from build123d import *

# Parameters (mm, degrees)
F1_DEPTH = 25


# Not quite as in the source:
# - a feature names something its author has since deleted; it is built from what else it names


with BuildPart() as f1:
    # F0 (on Top) → F1 (new body)
    with BuildSketch(Plane.XY):
        with BuildLine():
            Line((12.25, 5.25), (12.25, -5.25))
            Line((12.25, -5.25), (17.25, -5.25))
            Line((17.25, -5.25), (17.25, 10.25))
            Line((17.25, 10.25), (-17.288029389, 10.25))
            add(Edge.make_bspline(
                [(-17.288029389, 10.25), (-33.9326616892, 3.4588538136), (-27.6432598671, -11.5939724111), (-20.8629015828, -23.4088676175)],
                knots=[0, 0, 0, 0, 33.6081495202, 33.6081495202, 33.6081495202, 33.6081495202], degree=3))
            ThreePointArc((-20.8629015828, -23.4088676175), (-18.8330680728, -21.5504075494), (-16.1829780698, -20.8080323883))
            ThreePointArc((-16.1829780698, -20.8080323883), (-15.6956355504, -20.8090410674), (-15.2100205721, -20.8500513288))
            Line((-15.2100205721, -20.8500513288), (-15.2100205721, 3.0333888489))
            Line((-15.2100205721, 3.0333888489), (-12.4874287694, 3.0333888489))
            Line((-12.4874287694, 3.0333888489), (-12.25, 5.25))
            Line((-12.25, 5.25), (12.25, 5.25))
        make_face()
        Polygon((-12.4874287694, 3.0333888489), (-12.25, 3.0333888489), (-12.25, 5.25), align=None)
        with BuildLine():
            ThreePointArc((-10.0197441457, -26.7353467643), (-10.6063091532, -24.1634313379), (-12.25, -22.1001601804))
            ThreePointArc((-12.25, -22.1001601804), (-13.5686599523, -21.3031901955), (-15.0480940947, -20.872725511))
            Line((-15.0480940947, -20.872725511), (-15.2100205721, -22.3844548448))
            Line((-15.2100205721, -22.3844548448), (-15.2100205721, -20.8500513288))
            ThreePointArc((-15.2100205721, -20.8500513288), (-15.6956355504, -20.8090410674), (-16.1829780698, -20.8080323883))
            ThreePointArc((-16.1829780698, -20.8080323883), (-18.8330680728, -21.5504075494), (-20.8629015828, -23.4088676175))
            ThreePointArc((-20.8629015828, -23.4088676175), (-17.691321516, -32.4063150838), (-10.0197441457, -26.7353467643))
        make_face()
    extrude(amount=F1_DEPTH)


solid = f1.part
Can you work these out from the model? Positions are in its coordinate system, mm. A direction names the side the tool comes from. Give positions to 0.01 mm unless a question says otherwise; leave off trailing zeros. Order: outer loops, then holes, each group sorted by start corner. A loop starts at its lowest first (then second) coordinate and runs counter-clockwise, first axis right, second up. Notation, with made-up numbers: M 13,11 L 51,11 A24 cw 51,21 Z; hole C 26,-24 d11. An arc over 180 degrees is marked long. One line per question, with ' | ' between items.
Item 1: I'm going to push flat-ended pins straight in: pin 1 Ø0.9 at (x, z) = (-14, 11) entering from -Y; pin 2 Ø10 at (x, y) = (-12.5, -5.5) entering from -Z; pin 3 Ø2.5 at (x, z) = (14.5, 9) entering from -Y; pin 4 Ø4 at (y, z) = (-23.5, 3) entering from +X. Where does each tip first touch, or does it pass through?
Answer block:
pin 1: stops at y = -32.47 | pin 2: stops at z = 0 | pin 3: stops at y = -5.25 | pin 4: stops at x = -10.15
Item 2: Suppose I cut it at B-B, the plane x = 8. Write out the boundary of the cut face in (y, z).
Answer block:
outline: M 5.25,0 L 10.25,0 L 10.25,25 L 5.25,25 Z
Item 3: We'd pull the mould along X, two halves only. Please class faces 1 (the face through (15, -5.25, 12)), 2 (the face through (12.25, 0, 12)), 3 (the face through (17.25, 2, 12)): released by +X, released by -X, zero draft, split by the parting line, or undercut.
Answer block:
face 1: zero draft | face 2: undercut | face 3: released by +X
Item 4: Please list where these lines run through material, in increasing order: L1, parallel to Y at x = 15, z = 6.25; L2, parallel to Y at x = -1, z = 10.75; L3, parallel to X at y = -2.5, z = 6.
Answer block:
L1: y = -5.25 to 10.25 | L2: y = 5.25 to 10.25 | L3: x = -27.85 to -15.21, 12.25 to 17.25
Item 5: For faces 4 (the face through (-12.25, 4, 12)), 5 (the face through (-16, -5, 0)), which set-ups out of +Z, -Z, +X, -X, +Y, -Y let a thin tool reach every point of the face, with its end or its side?
Answer block:
face 4: +Z, -Z | face 5: -Z, +X, -X, +Y, -Y
Item 6: Suppose I cut it at A-A, the plane x = 13. Write out the boundary of the cut face in (y, z), then the cut area to 4 significant figures.
Answer block:
outline: M -5.25,0 L 10.25,0 L 10.25,25 L -5.25,25 Z | area: 387.5 mm2
